from build123d import *

# Parameters (mm, degrees)
F1_DEPTH = 600
F2_T     = -10
F5_DEPTH = 10


# Not quite as in the source:
# - a feature names something its author has since deleted; it is built from what else it names


with BuildPart() as f1:
    # F0 (on Top) → F1 (new body)
    with BuildSketch(Plane.XY):
        Polygon((-250, -250), (250, -250), (250, 250), (-50, 250), (-50, 50), (-250, 50), align=None)
    extrude(amount=F1_DEPTH)

    # F2
    f2_openings = [f1.faces().sort_by_distance(p)[0] for p in [
        (28.571429, -28.571429, 600),
    ]]
    offset(amount=F2_T, openings=f2_openings, kind=Kind.INTERSECTION)

    # F4 (on offset) → F5 (join)
    with BuildSketch(Plane.XY.offset(410)):
        Polygon((-240, 40), (-240, -240), (240, -240), (240, 240), (-40, 240), (-40, 40), align=None)
    extrude(amount=F5_DEPTH)


solid = f1.part
Design review of the part built by this model. Coordinates are the model's own, in mm. A direction names the side the tool comes from. Coordinates: 2 decimals unless noted, no trailing zeros. Loops run counter-clockwise (first coordinate to the right, second up) from the corner with the lowest first, then second, coordinate; pieces in that order, holes last. Notation, with made-up numbers: (21.25, 49.25) -> (49.25, 49.25) arc R11 ccw to (49.25, 69.25) -> close; hole circle Ø10 at (31.25, 28.25). An arc over 180 degrees is marked (long way). Use a Markdown table: item, result. Add a question column.
Item 1: The part is to be moulded in two halves that separate along X. For faces 1 (the flat face through (-149, 50, 296)), 2 (the flat face through (-50, 151, 296)), 3 (the flat face through (-240, -98, 207)), 4 (the flat face through (50, -50, 10)), say which applies: +X half, -X half, draft (parallel to the pull), parting line (faces both ways), or undercut.
Item 2: We need section A-A, the plane x = 49. Write out the cut boundary in (y, z).
Item 3: Machinability: for faces 5 (the flat face through (-242, 38, 600)), 6 (the flat face through (-139, 40, 509)), 7 (the flat face through (50, -50, 410)), which of the approach directions +Z, -Z, +X, -X, +Y, -Y give a long, thin tool a straight path to every point of the face, cutting with its end or side? Answer none if there is none.
Item 4: Clearance check with flat-ended pins moving along their axes: P1, Ø1.5, axis at x = -124.5, z = 414, coming from the +Y side; P2, Ø8, axis at x = -21, y = -1, coming from the +Z side. State where each tip first meets the part, or that it passes through.
Item 5: Wall thickness on L1, parallel to Z at x = 15, y = 197; L2, parallel to X at y = -152, z = 126: over which ranges is each line inside the solid? List them lowest first. Write a range as from..to.
Numbers:
| question | item | result |
|---|---|---|
| 1 | face 1 | draft |
| 1 | face 2 | -X half |
| 1 | face 3 | undercut |
| 1 | face 4 | undercut |
| 2 | outline | (-250, 0) -> (250, 0) -> (250, 600) -> (240, 600) -> (240, 420) -> (-240, 420) -> (-240, 600) -> (-250, 600) -> close; hole (-240, 10) -> (240, 10) -> (240, 410) -> (-240, 410) -> close |
| 3 | face 5 | +Z, +X, -X, +Y, -Y |
| 3 | face 6 | +Z |
| 3 | face 7 | none |
| 4 | P1 | stops at y = 50 |
| 4 | P2 | stops at z = 420 |
| 5 | L1 | z = 0..10, 410..420 |
| 5 | L2 | x = -250..-240, 240..250 |
